Design review of the part shown in the three views and the two pictorial views. Dimensions are in mm from the part's minimum x, y and z. Give positions to 0.01 mm unless a question says otherwise; leave off trailing zeros. Order: outer loops, then holes, each group sorted by start corner. A loop starts at its lowest first (then second) coordinate and runs counter-clockwise, first axis right, second up. Notation, with made-up numbers: M 33,75 L 68,75 A18 cw 68,104 Z; hole C 73,77 d6. An arc over 180 degrees is marked long. Answer as a JSON object with one key per item and string values.
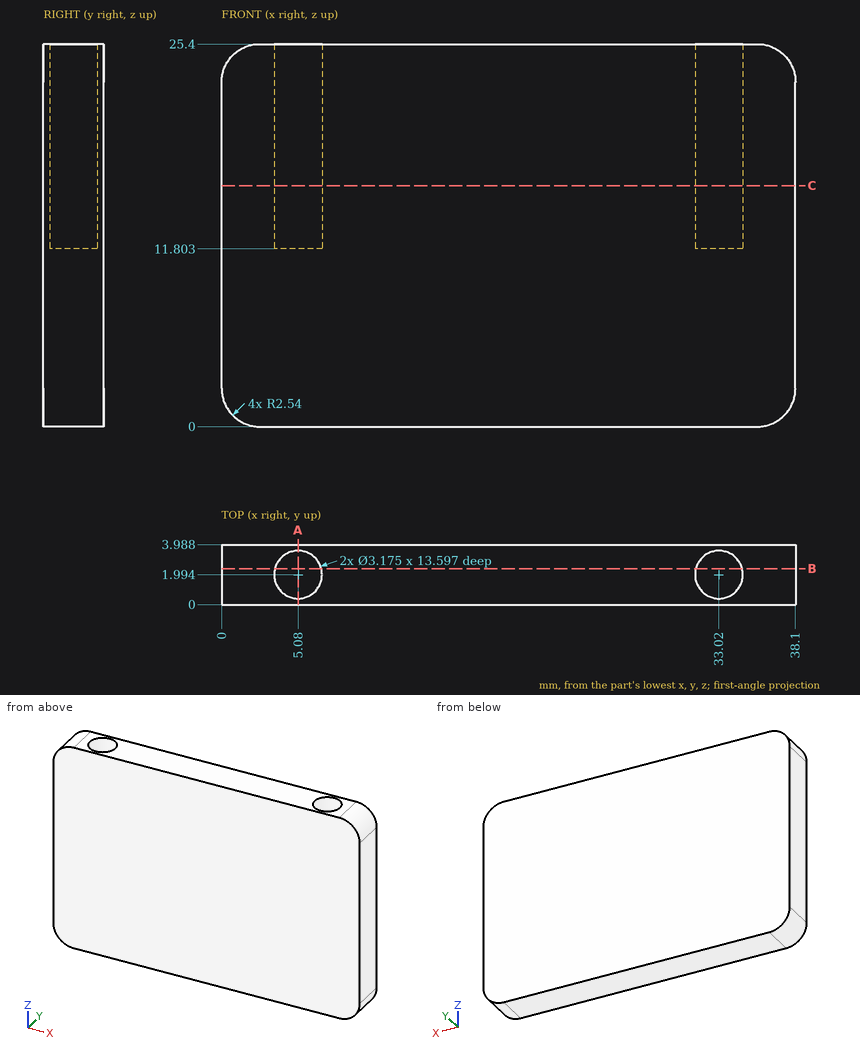
(1) We need section C-C (z = 16). Write out the cut boundary in (x, y) (1 decimal), plus the area to 3 significant figures.
Checked values:
{"outline": "M 0,0 L 38.1,0 L 38.1,4 L 0,4 Z; hole C 5.1,2 d3.2; hole C 33,2 d3.2", "area": "136 mm^2"}
(2) Insertion check: pin 1 (1.9 mm diameter, centred on x = 33.02, y = 1.99, fed in from +Z). The pin has a flat end and moves straight along its axis. Give the tip position at first contact, or say it passes through.
Checked values:
{"pin 1": "stops at z = 11.8"}
(3) To check wall thickness, follow L1, parallel to Y at x = 5.08, z = 21.5; L2, parallel to X at y = 2.8, z = 22.5; L3, parallel to X at y = 3.05, z = 18.75 (1 decimal). State the ranges of each line that lie inside material, in increasing order. Write a range as from..to.
Checked values:
{"L1": "y = 0..0.41, 3.58..3.99", "L2": "x = 0..3.71, 6.45..31.65, 34.39..38.1", "L3": "x = 0..3.9, 6.3..31.8, 34.2..38.1"}
(4) We need section A-A (x = 5.08). Write out the cut boundary in (y, z).
Checked values:
{"outline": "M 0,0 L 3.99,0 L 3.99,25.4 L 3.58,25.4 L 3.58,11.8 L 0.41,11.8 L 0.41,25.4 L 0,25.4 Z"}
(5) We need section B-B (y = 2.4). Write out the cut boundary in (x, z) (1 decimal).
Checked values:
{"outline": "M 0,2.5 A2.5 ccw 2.5,0 L 35.6,0 A2.5 ccw 38.1,2.5 L 38.1,22.9 A2.5 ccw 35.6,25.4 L 34.6,25.4 L 34.6,11.8 L 31.5,11.8 L 31.5,25.4 L 6.6,25.4 L 6.6,11.8 L 3.5,11.8 L 3.5,25.4 L 2.5,25.4 A2.5 ccw 0,22.9 Z"}
